Design review of the part built by this model. Coordinates are the model's own, in mm. A direction names the side the tool comes from. Give positions to 0.01 mm unless a question says otherwise; leave off trailing zeros. Write each loop counter-clockwise with the first axis right and the second up, starting at its lowest first coordinate (ties: lowest second). Pieces come first, ordered by that corner, then holes. Notation, with made-up numbers: (69, 1.25) -> (114, 1.25) arc R25 cw to (114, 27.25) -> close; hole circle Ø2 at (71, 48). An arc over 180 degrees is marked (long way). Answer as a JSON object with one key per item and string values.
Autodesk Inventor part; units mm, degrees
ref_plane "YZ Plane" through (0, 0, 0) normal (1, 0, 0) x (0, 1, 0)
ref_plane "XZ Plane" through (0, 0, 0) normal (0, 1, 0) x (-1, 0, 0)
ref_plane "XY Plane" through (0, 0, 0) normal (0, 0, 1) x (1, 0, 0)
sketch "Skizze1" plane through (0, 0, 0) normal (0, 1, 0) x (-1, 0, 0)
  circle A0 centre (0, 0) radius 3.22
  dimension "d0" = 6.44
extrude "Extrusion1" add sketch "Skizze1" along normal blind 47.6
sketch "Skizze2" plane through (0, 47.6, 0) normal (0, 1, 0) x (1, 0, 0)
  circle A0 centre (0, 0) radius 3.22
  circle A1 centre (0, 0) radius 3.22
  circle A2 centre (0, 0) radius 2.05
  dimension "d3" = 4.1
extrude "Extrusion2" add sketch "Skizze2" along normal blind 8.5 contours A2
sketch "Skizze3" plane through (0, 0, 0) normal (0, -1, 0) x (1, 0, 0)
  circle A0 centre (0, 0) radius 3.22
  ellipse E0 centre (0, 0) end of major axis (0, -9.5) minor radius 5.25
  line L0 (0, 9.5) -> (0, 0)
  line L1 (0, -10.6353) -> (0, 10.6353)
  line L2 (0, 0) -> (-5.25, 0)
  dimension "d6" = 9.5
  dimension "d7" = 5.25
extrude "Extrusion3" add sketch "Skizze3" along normal blind 1.5
sketch "Skizze4" plane through (0, -1.5, 0) normal (0, -1, 0) x (1, 0, 0)
  circle A0 centre (0, 0) radius 3.22
  circle A1 centre (0, 0) radius 2.165
  dimension "d10" = 4.33
extrude "Extrusion4" add sketch "Skizze4" along normal blind 9.5 contours A1
sketch "Skizze5" plane through (0, -11, 0) normal (0, -1, 0) x (1, 0, 0)
  circle A0 centre (0, 0) radius 2.165
  circle A1 centre (0, 0) radius 4.3
  dimension "d13" = 8.6
extrude "Extrusion5" add sketch "Skizze5" along normal blind 1.2 contours A0 | A1
sketch "Skizze6" plane through (0, -12.2, 0) normal (0, -1, 0) x (1, 0, 0)
  ellipse E0 centre (0, 0) end of major axis (0, -9.5) minor radius 5.25
  circle A0 centre (0, 0) radius 0.5
  dimension "d16" = 1
extrude "Extrusion6" add sketch "Skizze6" along normal blind 68.2 contours A0
sketch "Skizze7" plane through (0, -80.4, 0) normal (0, -1, 0) x (1, 0, 0)
  circle A0 centre (0, 0) radius 2.165
extrude "Extrusion7" add sketch "Skizze7" along normal blind 1.2
properties part number "00_Syringe_10ml"
(1) Clearance check with flat-ended pins moving along their axes: pin 1 (3 mm diameter, centred on x = -4, z = -6.5, fed in from +Y); pin 2 (5 mm diameter, centred on x = -1.5, z = 5, fed in from +Y); pin 3 (6 mm diameter, centred on x = 0, z = -4.5, fed in from +Y); pin 4 (8 mm diameter, centred on y = -54.5, z = -1.5, fed in from -X). State where each tip first meets the part, or that it passes through.
Here are the results:
{"pin 1": "stops at y = 0", "pin 2": "stops at y = 47.6", "pin 3": "stops at y = 56.1", "pin 4": "stops at x = -0.5"}
(2) The part is to be moulded in two halves that separate along Y. For faces 1 (the cylindrical face through (-1.718, -6.184, 1.317)), 2 (the flat face through (2, -11, -2)), 3 (the cylindrical face through (-1.718, -80.992, 1.317)), 4 (the flat face through (0, 56.1, 0)), say which applies: +Y half, -Y half, draft (parallel to the pull), parting line (faces both ways), or undercut.
Here are the results:
{"face 1": "undercut", "face 2": "undercut", "face 3": "draft", "face 4": "+Y half"}
(3) For faces 5 (the cylindrical face through (-4.296, -11.592, -0.189)), 6 (the flat face through (0, -81.6, 0)), 7 (the flat face through (-1, 47.6, -2)), list the 3-axis set-ups (+Z, -Z, +X, -X, +Y, -Y) from which the entire face can be reached by the end or side of a thin tool; tool diameter is ignored.
Here are the results:
{"face 5": "-Y", "face 6": "+Z, -Z, +X, -X, -Y", "face 7": "+Y"}
(4) For line 1 along Y through (x, z) = (-3, 0.25); line 2 along Y through (x, z) = (-0.75, -1.25); line 3 along Y through (x, z) = (-0.25, 6), list the stretches that pass through material, from the lowest coordinate up.
Here are the results:
{"line 1": "y = -12.2 to -11, -1.5 to 47.6", "line 2": "y = -81.6 to -80.4, -12.2 to 56.1", "line 3": "y = -1.5 to 0"}
(5) We need section A-A, the plane y = -59.5. State the section outline as (x, z) points, then the cut area to 3 significant figures.
Here are the results:
{"outline": "circle Ø1 at (0, 0)", "area": "0.785 mm²"}
(6) We need section B-B, the plane y = 2. State the section outline as (x, z) points, then the cut area to 3 significant figures.
Here are the results:
{"outline": "circle Ø6.44 at (0, 0)", "area": "32.6 mm²"}
